Geometry check sheet. Reference: the model listing, model coordinates, mm. A direction names the side the tool comes from. Coordinates: 2 decimals unless noted, no trailing zeros. Loops run counter-clockwise (first coordinate to the right, second up) from the corner with the lowest first, then second, coordinate; pieces in that order, holes last.
from build123d import *

# Parameters (mm, degrees)
SKETCH1_R           = 2
BOSS_EXTRUDE1_DEPTH = 5
BOSS_EXTRUDE2_START = -5
SKETCH3_R           = 5
SKETCH3_R_2         = 2
BOSS_EXTRUDE2_DEPTH = 5
SKETCH4_W           = 13.002851436
SKETCH4_H           = 2
CUT_EXTRUDE1_DEPTH  = 3
FILLET1_R           = 1
CUT_EXTRUDE2_START  = 2
SKETCH5_R           = 5
CUT_EXTRUDE2_DEPTH  = 2
FILLET2_R           = 1.5


with BuildPart() as part:
    # Sketch1 → Boss-Extrude1 (new body)
    with BuildSketch(Plane.XY):
        with BuildLine():
            Line((2, 0), (13, 0))
            ThreePointArc((13, 0), (0, 13), (-13, 0))
            ThreePointArc((-13, 0), (-5.5, -7.5), (2, 0))
        make_face()
        with Locations((-5.5, 0)):
            Circle(SKETCH1_R, mode=Mode.SUBTRACT)
    extrude(amount=BOSS_EXTRUDE1_DEPTH)

    # Sketch3 → Boss-Extrude2 (add)
    with BuildSketch(Plane.XY.offset(BOSS_EXTRUDE2_START)):
        with Locations((-5.5, 0)):
            Circle(SKETCH3_R)
        with Locations((-5.5, 0)):
            Circle(SKETCH3_R_2, mode=Mode.SUBTRACT)
    extrude(amount=BOSS_EXTRUDE2_DEPTH)

    # Sketch4 → Cut-Extrude1 (cut)
    with BuildSketch(Plane(origin=(0, 0, -5), x_dir=(-1, 0, 0), z_dir=(0, 0, -1))):
        with Locations((5.5, 0)):
            Rectangle(SKETCH4_W, SKETCH4_H)
    extrude(amount=-CUT_EXTRUDE1_DEPTH, mode=Mode.SUBTRACT)

    # Fillet1
    fillet1_edges = [part.edges().sort_by_distance(p)[0] for p in [
        (-8.815515147, 1, -2),
        (-2.184484853, 1, -2),
        (-8.815515147, -1, -2),
        (-2.184484853, -1, -2),
    ]]
    fillet(fillet1_edges, radius=FILLET1_R - 0.0001)  # a hair under: the kernel refuses the full size

    # Sketch5 → Cut-Extrude2 (cut)
    with BuildSketch(Plane(origin=(0, 0, 5), x_dir=(-1, 0, 0), z_dir=(0, 0, -1)).offset(CUT_EXTRUDE2_START)):
        with Locations(Location((5.5, 0, 0), (0, 0, 180))):
            Circle(SKETCH5_R)
    extrude(amount=-CUT_EXTRUDE2_DEPTH, mode=Mode.SUBTRACT)

    # Fillet2
    fillet2_edges = [part.edges().sort_by_distance(p)[0] for p in [
        (-10.5, 0, 0),
    ]]
    fillet(fillet2_edges, radius=FILLET2_R)


solid = part.part
(1) Sectioned sample at D-D on y = 7. Record the cut outline in (x, z).
Findings:
outline: (-10.95, 0) - (10.95, 0) - (10.95, 5) - (-10.95, 5) - close
(2) Sectioned sample at B-B on z = 4.25. Record the cut outline in (x, y), and give its area (3 significant figures).
Findings:
outline: (-13, 0) arc R7.5 ccw to (2, 0) - (13, 0) arc R13 ccw to start; hole circle Ø10 at (-5.5, 0)
area: 275 mm2
(3) Sectioned sample at A-A on x = -5.5. Record the cut outline in (y, z), and give its area (3 significant figures).
Findings:
outline: (-7.5, 0) - (-6.5, 0) arc R1.5 cw to (-5, -1.5) - (-5, -5) - (-2, -5) - (-2, 3) - (-5, 3) - (-5, 5) - (-7.5, 5) - close; (2, -5) - (5, -5) - (5, -1.5) arc R1.5 cw to (6.5, 0) - (11.78, 0) - (11.78, 5) - (5, 5) - (5, 3) - (2, 3) - close
area: 95.4 mm2
(4) Access from +Z, -Z, +X, -X, +Y, -Y to the whole of each face (thin tool, end or side, straight path). Record for faces 1 (the cylindrical face through (-0.73, 1.5, -3.27)), 2 (the flat face through (7, 0, 2)), 3 (the flat face through (-9, 1, -4)), 4 (the flat face through (-3, 0, 3)).
Findings:
face 1: -Z
face 2: +Z, -Z, +X, -Y
face 3: -Z, +X, -X
face 4: +Z
(5) Sectioned sample at C-C on x = 5. Record the cut outline in (y, z), and give its area (3 significant figures).
Findings:
outline: (0, 0) - (12, 0) - (12, 5) - (0, 5) - close
area: 60.0 mm2
(6) Gauge pin test, flat ends, axial feed: pin 1 Ø4 at (x, z) = (7.5, 1.5) entering from -Y; pin 2 Ø0.6 at (x, z) = (-9.5, -4) entering from -Y; pin 3 Ø2 at (x, z) = (-2.5, -4) entering from +Y; pin 4 Ø2.5 at (x, y) = (-5.5, 0) entering from +Z. Record the tip position at first contact, or that the pin passes through.
Findings:
pin 1: stops at y = 0
pin 2: stops at y = -3.36
pin 3: stops at y = 4.58
pin 4: passes through
(7) Scan lines: L1, parallel to X at y = 0, z = -1.75; L2, parallel to Y at x = -5.5, z = -2.5; L3, parallel to Z at x = 2.5, y = 6.25. Record each from-to range of solid material in increasing order.
Findings:
L1: x = -10.5 to -7.5, -3.5 to -0.5
L2: y = -5 to -2, 2 to 5
L3: z = 0 to 5
